Autodesk Inventor part; units mm, degrees
ref_plane "YZ Plane" through (0, 0, 0) normal (1, 0, 0) x (0, 1, 0)
ref_plane "XZ Plane" through (0, 0, 0) normal (0, 1, 0) x (-1, 0, 0)
ref_plane "XY Plane" through (0, 0, 0) normal (0, 0, 1) x (1, 0, 0)
sketch "Эскиз1" plane through (0, 0, 0) normal (0, 0, 1) x (1, 0, 0)
  circle A0 centre (0, 0) radius 5 construction
  circle A1 centre (0, 0) radius 1.575
  line L0 (343.1024, 82) -> (-136.8976, 82) construction
  line L1 (0, -5) -> (0, 110) construction
  line L2 (10, 5) -> (10, 100)
  line L3 (-10, 100) -> (-10, 5)
  arc A2 (-10, 5) -> (10, 5) centre (0, 5) ccw
  arc A3 (10, 100) -> (-10, 100) centre (0, 100) ccw
  circle A4 centre (0, 100) radius 1.575
  point P0 (0, 0)
  point P1 (0, 52.5)
  dimension "d0" = 115
  dimension "d1" = 20
extrude "Выдавливание1" add sketch "Эскиз1" along normal blind 10
properties part number "шатун"
The listing builds one solid part. Answer for the finished solid, in the listing's coordinates (mm). Round coordinates to 2 decimals unless told otherwise and drop trailing zeros. Loops run counter-clockwise (first coordinate to the right, second up) from the corner with the lowest first, then second, coordinate; pieces in that order, holes last.
Q1. Find the intervals of material crossed by line 1 (Y direction, x = 0, z = 2.5) (3 decimals); line 2 (X direction, y = 100, z = 7.25) (3 decimals); line 3 (Y direction, x = -8.25, z = 1.5), in increasing order.
Q2. For a pull along Y with two mould halves and no side action, classify faces 1 (the face through (0, -5, 5)), 2 (the face through (0, 110, 5)), 3 (the face through (-1.25, 0.96, 4.93)) as released by +Y, released by -Y, zero draft, split by the parting line, or undercut.
Q3. Section A-A, the plane x = 0 is taken. Determine the outline of the cut face in (y, z) (3 decimals), then the cut area to 3 significant figures.
Q4. Section B-B, the plane z = 8 is taken. Determine the outline of the cut face in (x, y) (3 decimals).
Q5. Given pin 1 Ø2 at (x, z) = (3.5, 1.5) entering from -Y; pin 2 Ø6 at (x, z) = (7, 5.5) entering from -Y; pin 3 Ø3 at (x, z) = (8, 4.5) entering from +Y, each flat-ended and moving along its own axis, determine where each tip first touches the part or whether it passes through.
Q6. Section D-D, the plane x = -5 is taken. Determine the outline of the cut face in (y, z).
Q7. Section C-C, the plane y = 0 is taken. Determine the outline of the cut face in (x, z) (3 decimals), then the cut area to 3 significant figures.
Completed:
1. line 1: y = -5 to -1.575, 1.575 to 98.425, 101.575 to 110
1. line 2: x = -10 to -1.575, 1.575 to 10
1. line 3: y = -0.65 to 105.65
2. face 1: released by -Y
2. face 2: released by +Y
2. face 3: undercut
3. outline: (-5, 0) - (-1.575, 0) - (-1.575, 10) - (-5, 10) - close; (1.575, 0) - (98.425, 0) - (98.425, 10) - (1.575, 10) - close; (101.575, 0) - (110, 0) - (110, 10) - (101.575, 10) - close
3. area: 1,090 mm2
4. outline: (-10, 5) arc R10 ccw to (10, 5) - (10, 100) arc R10 ccw to (-10, 100) - close; hole circle Ø3.15 at (0, 0); hole circle Ø3.15 at (0, 100)
5. pin 1: stops at y = -4.68
5. pin 2: stops at y = -4.17
5. pin 3: stops at y = 107.6
6. outline: (-3.66, 0) - (108.66, 0) - (108.66, 10) - (-3.66, 10) - close
7. outline: (-8.66, 0) - (-1.575, 0) - (-1.575, 10) - (-8.66, 10) - close; (1.575, 0) - (8.66, 0) - (8.66, 10) - (1.575, 10) - close
7. area: 142 mm2
